Autodesk Inventor part; units mm, degrees
ref_plane "Work Plane1" through (37.3126, 0, 0) normal (1, 0, 0) x (0, 0, -1)
ref_plane "Work Plane2" through (3.175, 0, 0) normal (-1, 0, 0) x (0, 0, 1)
ref_plane "YZ Plane" through (0, 0, 0) normal (1, 0, 0) x (0, 1, 0)
sketch "Sketch1" plane through (0, 0, 0) normal (1, 0, 0) x (0, 1, 0)
  circle A0 centre (0, 0) radius 3.175
  dimension "d0" = 6.35
extrude "Extrusion1" add sketch "Sketch1" along normal blind 40.4876
chamfer "Chamfer1" distance 0.508 angle 45 2 edges at (40.4876, -3.175, 0) (0, -3.175, 0)
ref_plane "Work Plane1" through (37.3126, 0, 0) normal (1, 0, 0) x (0, 0, -1)
sketch "Sketch2" plane through (37.3126, 0, 0) normal (1, 0, 0) x (0, 0, -1)
  circle A0 centre (0, 0) radius 2.3813
  circle A1 centre (0, 0) radius 3.175
  dimension "d7" = 4.7625
extrude "Extrusion2" cut sketch "Sketch2" along normal blind 1.5875
ref_plane "Work Plane2" through (3.175, 0, 0) normal (-1, 0, 0) x (0, 0, 1)
sketch "Sketch3" plane through (3.175, 0, 0) normal (-1, 0, 0) x (0, 0, 1)
  circle A0 centre (0, 0) radius 2.3813
  circle A1 centre (0, 0) radius 3.175
  dimension "d11" = 4.7625
extrude "Extrusion3" cut sketch "Sketch3" along normal blind 1.5875
properties part number "handle pivot pin"
For this review, take the finished solid that the model builds, in its own axes (mm). A direction names the side the tool comes from. Coordinates: 2 decimals unless noted, no trailing zeros. Loops run counter-clockwise (first coordinate to the right, second up) from the corner with the lowest first, then second, coordinate; pieces in that order, holes last. Notation, with made-up numbers: (3, 5.5) -> (22, 5.5) arc R21 ccw to (22, 23.5) -> close; hole circle Ø11 at (40, 60.25). An arc over 180 degrees is marked (long way). Return JSON: item names as keys, results as strings. Group by question number.
(1) Consider section C-C, the plane x = 6. Give the boundary of the cut face in (y, z) (3 decimals), plus the area to 3 significant figures.
(2) Consider section A-A, the plane y = 0. Give the boundary of the cut face in (x, z) (1 decimal).
(3) Mouldability with a two-part tool opening along X and no side actions: class faces 1 (the cylindrical face through (1.04, -0.69, 3.1)), 2 (the flat face through (40.488, 0, 0)), 3 (the cylindrical face through (38.1, 2.11, -1.1)) as pulls with the +X half, pulls with the -X half, needs draft (parallel to the pull), parting line crosses it, or undercut.
(4) To check wall thickness, follow L1, parallel to X at y = -2.25, z = -2 (1 decimal); L2, parallel to X at y = 2, z = -2 (1 decimal); L3, parallel to Y at x = 38, z = 1.25. State the ranges of each line that lie inside material, in increasing order.
(5) Tool access review of faces 4 (the flat face through (0, 0, 0)), 5 (the cylindrical face through (2.39, 2.11, 1.1)): name each direction out of +Z, -Z, +X, -X, +Y, -Y from which nothing blocks a thin tool from reaching the whole face with its end or side.
(6) For pin 1 Ø2 at (y, z) = (0, 0.5) entering from -X, flat-tipped, find the tip position at first contact; note if it passes through.
Results below:
{
 "1": {"outline": "circle Ø6.35 at (0, 0)", "area": "31.7 mm2"},
 "2": {"outline": "(0, -2.7) -> (0.5, -3.2) -> (1.6, -3.2) -> (1.6, -2.4) -> (3.2, -2.4) -> (3.2, -3.2) -> (37.3, -3.2) -> (37.3, -2.4) -> (38.9, -2.4) -> (38.9, -3.2) -> (40, -3.2) -> (40.5, -2.7) -> (40.5, 2.7) -> (40, 3.2) -> (38.9, 3.2) -> (38.9, 2.4) -> (37.3, 2.4) -> (37.3, 3.2) -> (3.2, 3.2) -> (3.2, 2.4) -> (1.6, 2.4) -> (1.6, 3.2) -> (0.5, 3.2) -> (0, 2.7) -> close"},
 "3": {"face 1": "needs draft", "face 2": "pulls with the +X half", "face 3": "undercut"},
 "4": {"L1": "x = 0.3 to 1.6, 3.2 to 37.3, 38.9 to 40.1", "L2": "x = 0.2 to 1.6, 3.2 to 37.3, 38.9 to 40.3", "L3": "y = -2.03 to 2.03"},
 "5": {"face 4": "+Z, -Z, -X, +Y, -Y", "face 5": "none"},
 "6": {"pin 1": "stops at x = 0"}
}
